```python
from build123d import *

# Parameters (mm, degrees)
FILLET1_R       = 0.1
RECPAT_COUNT    = 2
RECPAT_ANGLE    = 90
BALAYAGE1_PITCH = 1


with BuildPart() as part:
    # BodySke → Base-Revolve (revolve)
    with BuildSketch(Plane.XY, mode=Mode.PRIVATE) as base_revolve_sk:
        with BuildLine():
            Line((1.3, 0.7), (1.3, 2.5))
            Line((1.3, 2.5), (1, 2.5))
            Line((1, 2.5), (1, 1.75))
            Line((1, 1.75), (0.620174425, 1.75))
            ThreePointArc((0.620174425, 1.75), (0.531980628, 1.726913525), (0.466409986, 1.663576159))
            ThreePointArc((0.466409986, 1.663576159), (0.118808019, 0.863861087), (0, 0))
            Line((0, 0), (11.3, 0))
            Line((11.3, 0), (9.376765806, 0.7))
            Line((9.376765806, 0.7), (1.3, 0.7))
        make_face()
    revolve(base_revolve_sk.sketch.rotate(Axis((-25.4, 0, 0), (1, 0, 0)), 90), axis=Axis((-25.4, 0, 0), (1, 0, 0)))

    # Fillet1
    fillet1_edges = [part.edges().sort_by_distance(p)[0] for p in [
        (1.3, 0, -0.7),
    ]]
    fillet(fillet1_edges, radius=FILLET1_R)

    # Sketch3 → Recess section 0
    with BuildSketch(Plane(origin=(0, 0, 0), x_dir=(0, 0, -1), z_dir=(1, 0, 0))):
        with BuildLine():
            Line((0.24, -1.05), (-0.24, -1.05))
            Line((-0.24, -1.05), (-0.24, 1.05))
            Line((-0.24, 1.05), (0.24, 1.05))
            Line((0.24, 1.05), (0.24, -1.05))
        make_face()
    # Sketch4 → Recess section 1
    with BuildSketch(Plane(origin=(1.42, 0, 0), x_dir=(0, 0, -1), z_dir=(1, 0, 0))):
        with BuildLine():
            Line((0.24, -0.342014235), (-0.24, -0.342014235))
            Line((-0.24, -0.342014235), (-0.24, 0.342014235))
            Line((-0.24, 0.342014235), (0.24, 0.342014235))
            Line((0.24, 0.342014235), (0.24, -0.342014235))
        make_face()
    recess = loft(mode=Mode.SUBTRACT)

    # RecPat: Recess ×2 about axis
    recpat_axis = Axis((0, 0, 0), (1, 0, 0))
    for i in range(1, RECPAT_COUNT):
        add(recess.rotate(recpat_axis, i * RECPAT_ANGLE / (RECPAT_COUNT - 1)), mode=Mode.SUBTRACT)

    # RecCorSke → RecessCore (revolve, cut)
    with BuildSketch(Plane.XY, mode=Mode.PRIVATE) as recesscore_sk:
        Polygon((0, 0), (0, 0.454796073), (1.42, 0.3555), (1.535508952, 0), align=None)
    revolve(recesscore_sk.sketch.rotate(Axis((-3.175, 0, 0), (1, 0, 0)), 13.894577695), axis=Axis((-3.175, 0, 0), (1, 0, 0)), mode=Mode.SUBTRACT)

    # Balayage1: the profile of Esquisse2 profile screwed along a right-hand helix of 7.25 turns, 8 arcs to a turn; built about Z, then put on its axis
    balayage1_z = Axis((0, 0, 0), (0, 0, 1))
    balayage1_corners = [(0.6997, 0, -0.080465142), (1, 0, 0), (0.6997, 0, 0.080465142)]
    with BuildLine(mode=Mode.PRIVATE) as balayage1_profile:
        Line(balayage1_corners[0], balayage1_corners[1])
        Line(balayage1_corners[1], balayage1_corners[2])
        Line(balayage1_corners[2], balayage1_corners[0])
    balayage1_cap = Face(balayage1_profile.wire())
    balayage1_turn_angles = [0, 22.5, 45, 67.5, 90, 112.5, 135, 157.5, 180, 202.5, 225, 247.5, 270, 292.5, 315, 337.5, 360]
    balayage1_turn_weights = [1, 0.9238795325112867, 1, 0.9238795325112867, 1, 0.9238795325112867, 1, 0.9238795325112867, 1, 0.9238795325112867, 1, 0.9238795325112867, 1, 0.9238795325112867, 1, 0.9238795325112867, 1]
    balayage1_turn_rails = [Edge.make_bspline([Vector(p[0], p[1], 0).rotate(balayage1_z, balayage1_turn_angles[k]) / balayage1_turn_weights[k] + Vector(0, 0, p[2] + BALAYAGE1_PITCH * balayage1_turn_angles[k] / 360) for k in range(17)], [0, 0, 0, 1, 1, 2, 2, 3, 3, 4, 4, 5, 5, 6, 6, 7, 7, 8, 8, 8], 2, balayage1_turn_weights) for p in balayage1_corners]
    balayage1_turn_sides = [Face.make_surface_from_curves(balayage1_turn_rails[p[0]], balayage1_turn_rails[p[1]]) for p in [(0, 1), (1, 2), (2, 0)]]
    balayage1_last_angles = [2520, 2542.5, 2565, 2587.5, 2610]
    balayage1_last_weights = [1, 0.9238795325112867, 1, 0.9238795325112731, 1]
    balayage1_last_rails = [Edge.make_bspline([Vector(p[0], p[1], 0).rotate(balayage1_z, balayage1_last_angles[k]) / balayage1_last_weights[k] + Vector(0, 0, p[2] + BALAYAGE1_PITCH * balayage1_last_angles[k] / 360) for k in range(5)], [0, 0, 0, 1, 1, 2, 2, 2], 2, balayage1_last_weights) for p in balayage1_corners]
    balayage1_last_sides = [Face.make_surface_from_curves(balayage1_last_rails[p[0]], balayage1_last_rails[p[1]]) for p in [(0, 1), (1, 2), (2, 0)]]
    balayage1 = Plane(origin=(1.8, 0, 0), x_dir=(0, -1, 0), z_dir=(1, 0, 0)) * Solid(Shell([*[p.moved(Location((0, 0, BALAYAGE1_PITCH * i))) for i in range(7) for p in balayage1_turn_sides], *balayage1_last_sides, balayage1_cap, balayage1_cap.rotate(balayage1_z, 2610).moved(Location((0, 0, BALAYAGE1_PITCH * 2610 / 360)))]))
    add(balayage1)


solid = part.part
```
Model file for the job. Use its own axes, mm. A direction names the side the tool comes from. Coordinates: 2 decimals unless noted, no trailing zeros. Order: outer loops, then holes, each group sorted by start corner. A loop starts at its lowest first (then second) coordinate and runs counter-clockwise, first axis right, second up. Notation, with made-up numbers: (-11, 36) - (3, 36) arc R26 ccw to (3, 57) - close; hole circle Ø1 at (3, 16). An arc over 180 degrees is marked (long way). Return JSON: item names as keys, results as strings. Group by question number.
1) Flat gauge pins, fed straight in: P1, Ø3, axis at y = -0.5, z = 2, coming from the -X side; P2, Ø1.5, axis at x = 6, y = 1.5, coming from the -Z side; P3, Ø2, axis at x = 6.5, z = 1.5, coming from the -Y side. Where does each tip first touch, or does it go through?
2) Saw through at A-A, the plane z = -2.1. Write the cut outline in (x, y), plus the area to 3 significant figures.
3) Probe line 1 (X direction, y = 0.65, z = 2.2); line 2 (Y direction, x = 0.5, z = -0.65); line 3 (X direction, y = -1.15, z = 0.15). List the from-to ranges inside material, lowest first. Write a range as from..to.
4) Saw through at C-C, the plane y = -1.9. Write the cut outline in (x, z), plus the area to 3 significant figures.
5) Tool access for faces 1 (the cylindrical face through (1.15, 2.22, 1.15)), 2 (the cylindrical face through (0.81, 1.55, 0.81)): list every direction of +Z, -Z, +X, -X, +Y, -Y with a clear straight run to the whole face (end or side of a thin tool).
6) Saw through at B-B, the plane x = 9.75. Write the cut outline in (y, z).
Values found:
{
 "1": {"P1": "stops at x = 0.05", "P2": "stops at z = -0.63", "P3": "stops at y = -0.85"},
 "2": {"outline": "(1, -1.36) - (1.3, -1.36) - (1.3, 1.36) - (1, 1.36) - close", "area": "0.814 mm²"},
 "3": {"line 1": "x = 1..1.3", "line 2": "y = -1.58..-0.24, 0.24..1.58", "line 3": "x = 0.22..1.3"},
 "4": {"outline": "(1, -1.62) - (1.3, -1.62) - (1.3, 1.62) - (1, 1.62) - close", "area": "0.975 mm²"},
 "5": {"face 1": "+X, -X", "face 2": "-X"},
 "6": {"outline": "circle Ø1.13 at (0, 0)"}
}
